Design review of the part built by this model. Coordinates are the model's own, in mm. Face numbers are marked on the shaded views. A direction names the side the tool comes from. Give positions to 0.01 mm unless a question says otherwise; leave off trailing zeros. Order: outer loops, then holes, each group sorted by start corner. A loop starts at its lowest first (then second) coordinate and runs counter-clockwise, first axis right, second up. Notation, with made-up numbers: (56.5, 14.5) -> (106.5, 14.5) arc R20 ccw to (106.5, 45.5) -> close; hole circle Ø3 at (19, -25.5). An arc over 180 degrees is marked (long way). One line per item, written item: value.
from build123d import *

# Parameters (mm, degrees)
SKETCH1_R                          = 4.375
SKETCH1_W                          = 0.93
SKETCH1_H                          = 10
BOSS_EXTRUDE1_DEPTH                = 30
SKETCH2_W                          = 8
SKETCH2_H                          = 26
BOSS_EXTRUDE3_DEPTH                = 1
FILLET4_R                          = 3
FILLET5_DEPTH                      = 25.878263471
FILLET5_START                      = 14.878263371
FILLET5_2_DEPTH                    = 11.0000001
FILLET5_START_2                    = -3
FILLET5_3_DEPTH                    = 2.07
CUT_EXTRUDE1_REACH                 = 37.895
SKETCH3_R                          = 0.5
SKETCH4_W                          = 10
SKETCH4_H                          = 2
BOSS_EXTRUDE4_DEPTH                = 30
CUT_EXTRUDE2_REACH                 = 39.004
SKETCH5_R                          = 3.875
CUT_EXTRUDE4_REACH                 = 39.004
M2_5X0_45_TAPPED_HOLE1_D           = 2.05
M2_5X0_45_TAPPED_HOLE1_CSINK_D     = 2.55
M2_5X0_45_TAPPED_HOLE1_CSINK_ANGLE = 90


with BuildPart() as part:
    # Sketch1 → Boss-Extrude1 (new body)
    with BuildSketch(Plane(origin=(0, 0, 0), x_dir=(0, 0, -1), z_dir=(1, 0, 0))):
        with Locations((4.805, 5)):
            Circle(SKETCH1_R)
        with Locations((0.465, 5)):
            Rectangle(SKETCH1_W, SKETCH1_H)
    extrude(amount=BOSS_EXTRUDE1_DEPTH)

    # Sketch2 → Boss-Extrude3 (add)
    with BuildSketch(Plane.XY):
        with Locations((21.878263471, 4.931133475)):
            Rectangle(SKETCH2_W, SKETCH2_H)
    extrude(amount=-BOSS_EXTRUDE3_DEPTH)

    # Fillet4
    fillet4_edges = [part.edges().sort_by_distance(p)[0] for p in [
        (17.878263471, 10, -0.465),
        (25.878263471, 10, -0.465),
        (17.878263471, 0, -0.465),
        (25.878263471, 0, -0.465),
    ]]
    fillet(fillet4_edges, radius=FILLET4_R)

    # Fillet5: read off the stored shape, not the designer's step
    # Fillet5 outline → Fillet5 (add)
    with BuildSketch(Plane.YZ):
        with BuildLine():
            ThreePointArc((9.344098712, -4.285932203), (9.442351653, -3.091914153), (10, -2.031555221))
            Line((10, -2.031555221), (10, -0.93))
            Line((10, -0.93), (7.031009601, -0.93))
            ThreePointArc((7.031009601, -0.93), (8.602231494, -2.32214816), (9.344098712, -4.285932203))
        make_face()
        with BuildLine():
            ThreePointArc((0, -2.031555221), (0.557648347, -3.091914153), (0.655901288, -4.285932203))
            ThreePointArc((0.655901288, -4.285932203), (1.397768506, -2.32214816), (2.968990399, -0.93))
            Line((2.968990399, -0.93), (0, -0.93))
            Line((0, -0.93), (0, -2.031555221))
        make_face()
    extrude(amount=FILLET5_DEPTH)

    # Fillet5 2 outline → Fillet5 2 (add)
    with BuildSketch(Plane.YZ.offset(FILLET5_START)):
        with BuildLine():
            ThreePointArc((10, -2.031555221), (11.037478267, -1.219341931), (12.322909258, -0.93))
            Line((12.322909258, -0.93), (10, -0.93))
            Line((10, -0.93), (10, -2.031555221))
        make_face()
        with BuildLine():
            Line((0, -2.031555221), (0, -0.93))
            Line((0, -0.93), (-2.322909258, -0.93))
            ThreePointArc((-2.322909258, -0.93), (-1.037478267, -1.219341931), (0, -2.031555221))
        make_face()
    extrude(amount=FILLET5_2_DEPTH)

    # Fillet5 3 outline → Fillet5 3 (cut)
    with BuildSketch(Plane.XY.offset(FILLET5_START_2)):
        with BuildLine():
            ThreePointArc((14.878263471, 10), (16.999583814, 10.878679656), (17.878263471, 13))
            Line((17.878263471, 13), (17.878263471, 14))
            Line((17.878263471, 14), (14.878263371, 14))
            Line((14.878263371, 14), (14.878263471, 10))
        make_face()
        with BuildLine():
            Line((14.878263371, -4), (17.878263471, -4))
            Line((17.878263471, -4), (17.878263471, -3))
            ThreePointArc((17.878263471, -3), (16.999583814, -0.878679657), (14.878263471, 0))
            Line((14.878263471, 0), (14.878263371, -4))
        make_face()
    extrude(amount=FILLET5_3_DEPTH, mode=Mode.SUBTRACT)

    # Sketch3 → Cut-Extrude1 (cut, up to next)
    with BuildSketch(Plane(origin=(0, 0, -1), x_dir=(-1, 0, 0), z_dir=(0, 0, -1)), mode=Mode.PRIVATE) as cut_extrude1_sk1:
        with Locations((-21.730165356, 13.098626711)):
            Circle(SKETCH3_R)
    cut_extrude1_tool1 = extrude(cut_extrude1_sk1.sketch, amount=-CUT_EXTRUDE1_REACH, mode=Mode.PRIVATE) & part.part
    # Sketch3 → Cut-Extrude1 (cut, up to next)
    with BuildSketch(Plane(origin=(0, 0, -1), x_dir=(-1, 0, 0), z_dir=(0, 0, -1)), mode=Mode.PRIVATE) as cut_extrude1_sk2:
        with Locations((-21.851713242, -3.100917298)):
            Circle(SKETCH3_R)
    cut_extrude1_tool2 = extrude(cut_extrude1_sk2.sketch, amount=-CUT_EXTRUDE1_REACH, mode=Mode.PRIVATE) & part.part
    add(cut_extrude1_tool1.solids().sort_by_distance((21.730165, 13.098627, -1))[0], mode=Mode.SUBTRACT)
    add(cut_extrude1_tool2.solids().sort_by_distance((21.851713, -3.100917, -1))[0], mode=Mode.SUBTRACT)

    # Sketch4 → Boss-Extrude4 (add)
    with BuildSketch(Plane(origin=(30, 0, 0), x_dir=(0, 0, -1), z_dir=(1, 0, 0))):
        with Locations((7.157056942, 4.926549366)):
            Rectangle(SKETCH4_W, SKETCH4_H)
    extrude(amount=-BOSS_EXTRUDE4_DEPTH)

    # Sketch5 → Cut-Extrude2 (cut, up to next)
    with BuildSketch(Plane(origin=(30, 0, 0), x_dir=(0, 0, -1), z_dir=(1, 0, 0)), mode=Mode.PRIVATE) as cut_extrude2_sk1:
        with Locations((4.815292967, 5.000024119)):
            Circle(SKETCH5_R)
    cut_extrude2_tool1 = extrude(cut_extrude2_sk1.sketch, amount=-CUT_EXTRUDE2_REACH, mode=Mode.PRIVATE) & part.part
    add(cut_extrude2_tool1.solids().sort_by_distance((30, 5.000024, -4.815293))[0], mode=Mode.SUBTRACT)

    # Sketch6 → Cut-Extrude4 (cut, up to next)
    with BuildSketch(Plane(origin=(30, 0, 0), x_dir=(0, 0, -1), z_dir=(1, 0, 0)), mode=Mode.PRIVATE) as cut_extrude4_sk1:
        with BuildLine():
            Line((12.157056942, 5.176549366), (12.157056942, 4.676549366))
            Line((12.157056942, 4.676549366), (8.676767955, 4.676549366))
            add(Edge.make_bspline(
                [(8.676767955, 4.676549366), (8.69766925, 4.926395918), (8.686270084, 5.176549366)],
                knots=[0, 0, 0, 1, 1, 1], degree=2))
            Line((8.686270084, 5.176549366), (12.157056942, 5.176549366))
        make_face()
    cut_extrude4_tool1 = extrude(cut_extrude4_sk1.sketch, amount=-CUT_EXTRUDE4_REACH, mode=Mode.PRIVATE) & part.part
    add(cut_extrude4_tool1.solids().sort_by_distance((30, 4.926435, -10.421978))[0], mode=Mode.SUBTRACT)

    # M2.5x0.45 Tapped Hole1 (through all)
    with Locations(Plane(origin=(0, 3.926549366, 0), x_dir=(-1, 0, 0), z_dir=(0, -1, 0))):
        with Locations((-25.5, 10.599323574), (-4.5, 10.599323574)):
            CounterSinkHole(M2_5X0_45_TAPPED_HOLE1_D / 2, M2_5X0_45_TAPPED_HOLE1_CSINK_D / 2, counter_sink_angle=M2_5X0_45_TAPPED_HOLE1_CSINK_ANGLE)


solid = part.part
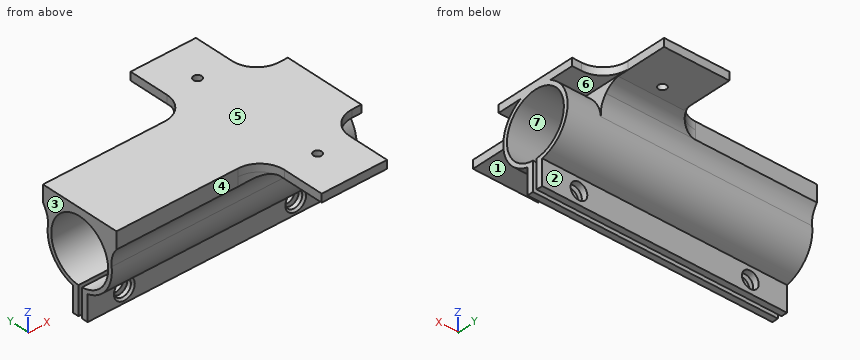
Item 1: Add section C-C on y = 16.75. Give the boundary of the cut face in (x, z), plus the area to 3 significant figures.
Returned:
outline: (17.88, -1) -> (25.88, -1) -> (25.88, 0) -> (17.88, 0) -> close
area: 8.00 mm²
Item 2: Add section D-D on x = 16.5. Give the boundary of the cut face in (y, z) (3 decimals), plus the area to 3 significant figures.
Returned:
outline: (-0.476, -1.566) arc R3 cw to (0.656, -4.286) arc R4.375 ccw to (3.927, -9.046) -> (3.927, -12.157) -> (4.677, -12.157) -> (4.677, -8.677) arc R3.875 cw (long way) to (5.177, -8.686) -> (5.177, -12.157) -> (5.927, -12.157) -> (5.927, -9.081) arc R4.375 ccw to (9.344, -4.286) arc R3 cw to (10.476, -1.566) -> (10.476, 0) -> (-0.476, 0) -> close
area: 34.0 mm²
Item 3: Clearance check with flat-ended pins moving along their axes: P1, Ø1, axis at x = 7, z = -1, coming from the +Y side; P2, Ø3.5, axis at x = 28, y = 0, coming from the -Z side; P3, Ø0.5, axis at y = 14.5, z = -0.5, coming from the -X side; P4, Ø6, axis at x = 10.5, y = -4.5, coming from the +Z side. State where each tip first meets the part, or that it passes through.
Returned:
P1: y = 10
P2: z = -7.73
P3: x = 17.88
P4: through
Item 4: Machinability: for the marked faces 1, 2 and 3, which of the approach directions +Z, -Z, +X, -X, +Y, -Y give a long, thin tool a straight path to every point of the face, cutting with its end or side? Answer none if there is none.
Returned:
face 1: -Z, +X, -X, -Y
face 2: -Z, +X, -X, +Y
face 3: +Z, -Z, -X, +Y, -Y
Item 5: To check wall thickness, follow line 1 along Y through (x, z) = (6.25, -9.75); line 2 along Z through (x, y) = (25.5, 4.3); line 3 along Z through (x, y) = (27, 1.5). State the ranges of each line that lie inside material, in increasing order. Write a range as from..to.
Returned:
line 1: 3.93..4.68, 5.18..5.93
line 2: -12.16..-11.62, -9.57..-8.63, -1..0
line 3: -7.43..-6.48, -3.15..-2.18, -0.93..0
Item 6: Add section A-A on z = -3. Give the boundary of the cut face in (x, y), plus the area to 3 significant figures.
Returned:
outline: (0, 0.53) -> (25.88, 0.53) -> (25.88, 1.01) -> (30, 1.01) -> (30, 1.58) -> (0, 1.58) -> close; (0, 8.42) -> (30, 8.42) -> (30, 8.99) -> (25.88, 8.99) -> (25.88, 9.47) -> (0, 9.47) -> close
area: 58.8 mm²
Item 7: Add section B-B on x = 4.5. Give the boundary of the cut face in (y, z) (3 decimals), plus the area to 3 significant figures.
Returned:
outline: (0, -2.032) arc R3 cw to (0.656, -4.286) arc R4.375 ccw to (3.927, -9.046) -> (3.927, -9.324) -> (4.177, -9.574) -> (4.677, -9.574) -> (4.677, -8.677) arc R3.875 cw (long way) to (5.177, -8.686) -> (5.177, -9.574) -> (5.927, -9.574) -> (5.927, -9.081) arc R4.375 ccw to (9.344, -4.286) arc R3 cw to (10, -2.032) -> (10, 0) -> (0, 0) -> close; (3.927, -12.157) -> (4.677, -12.157) -> (4.677, -11.624) -> (4.177, -11.624) -> (3.927, -11.874) -> close; (5.177, -12.157) -> (5.927, -12.157) -> (5.927, -11.624) -> (5.177, -11.624) -> close
area: 29.2 mm²
Item 8: Draft analysis for pull direction Z (two halves, no side actions). For the marked faces 4, 5, 6 and 7, state which applies: pulls with the +Z half, pulls with the -Z half, needs draft (parallel to the pull), parting line crosses it, or undercut.
Returned:
face 4: needs draft
face 5: pulls with the +Z half
face 6: undercut
face 7: undercut
